The listing builds one solid part. Answer for the finished solid, in the listing's coordinates (mm). A direction names the side the tool comes from. Coordinates: 2 decimals unless noted, no trailing zeros. Order: outer loops, then holes, each group sorted by start corner. A loop starts at its lowest first (then second) coordinate and runs counter-clockwise, first axis right, second up. Notation, with made-up numbers: (80.5, -18) -> (98.5, -18) arc R12 ccw to (98.5, -3) -> close; hole circle Ø1 at (7.5, -7). An arc over 180 degrees is marked (long way). Write each question's results on one line, items separated by ' | '. Start each with the question number.
(1) Determine the mould class of faces 4 (the face through (71, 84, 50)), 5 (the face through (67, 35, 60)), 6 (the face through (58.794, 37.492, 59.572)) for opening direction Y: +Y half, -Y half, draft (parallel to the pull), parting line (faces both ways), or undercut.
(2) The part is cut by section D-D, the plane y = 38.8. Give the vertices of the cut face in (x, z), then the cut area to 3 significant figures.
(3) Straight lines are drawn through the part: L1, parallel to X at y = 38.8, z = 60.1; L2, parallel to Z at x = 73.5, y = 42.5; L3, parallel to Y at x = 60.5, z = 41.2. For each, find the intervals that lie inside material, in ascending order.
(4) The part is cut by section B-B, the plane x = 69.5. Give the vertices of the cut face in (y, z).
(5) The part is cut by section C-C, the plane z = 50. Give the vertices of the cut face in (x, y), then the cut area to 3 significant figures.
(6) A tool of negligible diameter and unlimited length cuts with its end or side. For faces 1 (the face through (69, 60, 61.6)), 2 (the face through (61, 45, 60)), 3 (the face through (71, 44, 50)), from which of +Z, -Z, +X, -X, +Y, -Y can it reach the whole face along a straight path? Write none if from no direction.
(7) The part is cut by section A-A, the plane y = 69. Give the vertices of the cut face in (x, z).
(8) Given pin 1 (12 mm diameter, centred on y = 69, z = 50.5, fed in from +X); pin 2 (6 mm diameter, centred on x = 72, z = 50, fed in from -Y); pin 3 (1.2 mm diameter, centred on x = 60, z = 59, fed in from +Y); pin 4 (4 mm diameter, centred on x = 60.5, y = 38.8, fed in from -Z), each flat-ended and moving along its own axis, determine where each tip first touches the part or whether it passes through.
```python
from build123d import *

# Parameters (mm, degrees)
GUIDED_START                               = 38.4
SKETCH1_W                                  = 12
SKETCH1_H                                  = 40
GUIDED_BRIDGE_WITH_ROD_COUPLING_SEAT_DEPTH = 23.2
LOWER_START                                = 38.4
SKETCH2_W                                  = 19
SKETCH2_H                                  = 10
LOWER_LAP_EAR_CLEARS_STOP_STATION_DEPTH    = 4
UPPER_START                                = 57.6
SKETCH3_W                                  = 19
SKETCH3_H                                  = 10
UPPER_LAP_EAR_CLEARS_STOP_STATION_DEPTH    = 4
M4_START                                   = 38.4
SKETCH4_R                                  = 2.15
M4_JOINT_BOLT_CLEARANCE_DEPTH              = 23.2
RADIAL_START                               = 65
SKETCH5_R                                  = 6.15
RADIAL_FLOATING_STUD_CLEARANCE_DEPTH       = 12


with BuildPart() as part:
    # Sketch1 → Guided bridge with rod coupling seat (new body)
    with BuildSketch(Plane.XY.offset(GUIDED_START)):
        with Locations((71, 64)):
            Rectangle(SKETCH1_W, SKETCH1_H)
    extrude(amount=GUIDED_BRIDGE_WITH_ROD_COUPLING_SEAT_DEPTH)

    # Sketch2 → Lower lap ear clears stop station (add)
    with BuildSketch(Plane.XY.offset(LOWER_START)):
        with Locations((67.5, 40)):
            Rectangle(SKETCH2_W, SKETCH2_H)
    extrude(amount=LOWER_LAP_EAR_CLEARS_STOP_STATION_DEPTH)

    # Sketch3 → Upper lap ear clears stop station (add)
    with BuildSketch(Plane.XY.offset(UPPER_START)):
        with Locations((67.5, 40)):
            Rectangle(SKETCH3_W, SKETCH3_H)
    extrude(amount=UPPER_LAP_EAR_CLEARS_STOP_STATION_DEPTH)

    # Sketch4 → M4 joint bolt clearance (cut)
    with BuildSketch(Plane.XY.offset(M4_START)):
        with Locations((60.5, 38.8)):
            Circle(SKETCH4_R)
        with Locations((69.5, 38.8)):
            Circle(SKETCH4_R)
    extrude(amount=M4_JOINT_BOLT_CLEARANCE_DEPTH, mode=Mode.SUBTRACT)

    # Sketch5 → Radial floating stud clearance (cut)
    with BuildSketch(Plane(origin=(0, 0, 0), x_dir=(0, 0, -1), z_dir=(1, 0, 0)).offset(RADIAL_START)):
        with Locations((-50, 69)):
            Circle(SKETCH5_R)
    extrude(amount=RADIAL_FLOATING_STUD_CLEARANCE_DEPTH, mode=Mode.SUBTRACT)


solid = part.part
```
Established:
1) face 4: +Y half | face 5: -Y half | face 6: undercut
2) outline: (58, 38.4) -> (58.35, 38.4) -> (58.35, 42.4) -> (58, 42.4) -> close; (58, 57.6) -> (58.35, 57.6) -> (58.35, 61.6) -> (58, 61.6) -> close; (62.65, 38.4) -> (67.35, 38.4) -> (67.35, 42.4) -> (62.65, 42.4) -> close; (62.65, 57.6) -> (67.35, 57.6) -> (67.35, 61.6) -> (62.65, 61.6) -> close; (71.65, 38.4) -> (77, 38.4) -> (77, 42.4) -> (71.65, 42.4) -> close; (71.65, 57.6) -> (77, 57.6) -> (77, 61.6) -> (71.65, 61.6) -> close | area: 83.2 mm^2
3) L1: x = 58 to 58.35, 62.65 to 67.35, 71.65 to 77 | L2: z = 38.4 to 42.4, 57.6 to 61.6 | L3: y = 35 to 36.65, 40.95 to 45
4) outline: (35, 38.4) -> (36.65, 38.4) -> (36.65, 42.4) -> (35, 42.4) -> close; (35, 57.6) -> (36.65, 57.6) -> (36.65, 61.6) -> (35, 61.6) -> close; (40.95, 38.4) -> (84, 38.4) -> (84, 61.6) -> (40.95, 61.6) -> (40.95, 57.6) -> (44, 57.6) -> (44, 42.4) -> (40.95, 42.4) -> close; hole circle Ø12.3 at (69, 50)
5) outline: (65, 44) -> (77, 44) -> (77, 62.85) -> (65, 62.85) -> close; (65, 75.15) -> (77, 75.15) -> (77, 84) -> (65, 84) -> close | area: 332 mm^2
6) face 1: +Z, +X, -X, +Y, -Y | face 2: +Z, -Z, -X, +Y | face 3: +X, -X, -Y
7) outline: (65, 38.4) -> (77, 38.4) -> (77, 43.85) -> (65, 43.85) -> close; (65, 56.15) -> (77, 56.15) -> (77, 61.6) -> (65, 61.6) -> close
8) pin 1: stops at x = 77 | pin 2: stops at y = 44 | pin 3: stops at y = 45 | pin 4: passes through
